The model under review builds one solid part; all positions refer to its coordinate system, in mm. Face numbers are marked on the shaded views. A direction names the side the tool comes from. Coordinates: 2 decimals unless noted, no trailing zeros. Loops run counter-clockwise (first coordinate to the right, second up) from the corner with the lowest first, then second, coordinate; pieces in that order, holes last. Notation, with made-up numbers: M -21.75,-10 L 21.25,-10 A5 cw 21.25,-4 Z; hole C 26,66 d4. An arc over 180 degrees is marked long. Use CSV: the item, a comma, the result in double quotes. Start each with the question number.
from build123d import *

# Parameters (mm, degrees)
BOSS_EXTRUDE1_DEPTH     = 24
FILLET1_R               = 14
CUT_EXTRUDE1_DEPTH      = 36
CUT_EXTRUDE1_DEPTH_BACK = 21


with BuildPart() as part:
    # Sketch1 → Boss-Extrude1 (new body, symmetric)
    with BuildSketch(Plane.XY):
        with BuildLine():
            Line((35, 0), (48, 0))
            Line((48, 0), (48, 6))
            Line((48, 6), (95, 6))
            Line((95, 6), (95, 20))
            Line((95, 20), (51.23475383, 20))
            ThreePointArc((51.23475383, 20), (0, 55), (-51.23475383, 20))
            Line((-51.23475383, 20), (-95, 20))
            Line((-95, 20), (-95, 6))
            Line((-95, 6), (-48, 6))
            Line((-48, 6), (-48, 0))
            Line((-48, 0), (-35, 0))
            ThreePointArc((-35, 0), (0, 35), (35, 0))
        make_face()
    extrude(amount=BOSS_EXTRUDE1_DEPTH, both=True)

    # Fillet1
    fillet1_edges = [part.edges().sort_by_distance(p)[0] for p in [
        (95, 13, -24),
        (-95, 13, -24),
        (95, 13, 24),
        (-95, 13, 24),
    ]]
    fillet(fillet1_edges, radius=FILLET1_R)

    # Sketch2 → Cut-Extrude1 (cut, two sides)
    with BuildSketch(Plane(origin=(0, 20, 0), x_dir=(1, 0, 0), z_dir=(0, 1, 0))) as cut_extrude1_sk:
        with BuildLine():
            Line((68, -7), (68, 13))
            ThreePointArc((68, 13), (75, 20), (82, 13))
            Line((82, 13), (82, -7))
            ThreePointArc((82, -7), (75, -14), (68, -7))
        make_face()
        with BuildLine():
            Line((-68, -7), (-68, 13))
            ThreePointArc((-68, 13), (-75, 20), (-82, 13))
            Line((-82, 13), (-82, -7))
            ThreePointArc((-82, -7), (-75, -14), (-68, -7))
        make_face()
    extrude(amount=CUT_EXTRUDE1_DEPTH, mode=Mode.SUBTRACT)
    extrude(cut_extrude1_sk.sketch, amount=-CUT_EXTRUDE1_DEPTH_BACK, mode=Mode.SUBTRACT)


solid = part.part
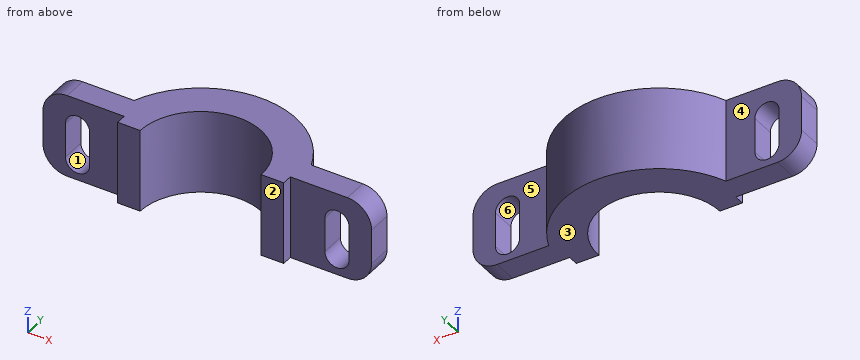
1. Add section D-D (y = 25.5). Write out the cut boundary in (x, z).
2. For the marked faces 4, 5 and 6, list the 3-axis set-ups (+Z, -Z, +X, -X, +Y, -Y) from which the entire face can be reached by the end or side of a thin tool; tool diameter is ignored.
3. Add section C-C (z = -16). Write out the cut boundary in (x, y).
4. Add section A-A (x = -75). Write out the cut boundary in (y, z), plus the area to 3 significant figures.
5. Draft analysis for pull direction Z (two halves, no side actions). For the marked faces 1, 2 and 3, state which applies: released by +Z, released by -Z, zero draft, split by the parting line, or undercut.
6. Insertion check: pin 1 Ø1 at (y, z) = (30.5, 0.5) entering from +X; pin 2 Ø1.5 at (y, z) = (37.5, -10.5) entering from -X; pin 3 Ø8 at (x, z) = (58.5, -3) entering from -Y. Each pin has a flat end and moves straight along its axis. Give the tip position at first contact, or say it passes through.
7. To check wall thickness, follow line 1 along X through (y, z) = (17.5, -2); line 2 along X through (y, z) = (15, -0.5); line 3 along Y through (x, z) = (84.5, -1). State the ranges of each line that lie inside material, in increasing order.
8. Add section B-B (y = 17). Write out the cut boundary in (x, z).
Solved:
1,outline,"M -48.73,-24 L -23.97,-24 L -23.97,24 L -48.73,24 Z; M 23.97,-24 L 48.73,-24 L 48.73,24 L 23.97,24 Z"
2,face 4,"+Z, -Z, -X, +Y"
2,face 5,"+Z, -Z, +X, +Y"
2,face 6,"+Y, -Y"
3,outline,"M -93.65,6 L -81.32,6 L -81.32,20 L -93.65,20 Z; M -68.68,6 L -48,6 L -48,0 L -35,0 A35 cw 35,0 L 48,0 L 48,6 L 68.68,6 L 68.68,20 L 51.23,20 A55 ccw -51.23,20 L -68.68,20 Z; M 81.32,6 L 93.65,6 L 93.65,20 L 81.32,20 Z"
4,outline,"M 6,-24 L 20,-24 L 20,-20 L 6,-20 Z; M 6,14 L 20,14 L 20,24 L 6,24 Z"
4,area,"196 mm^2"
5,face 1,"undercut"
5,face 2,"zero draft"
5,face 3,"released by -Z"
6,pin 1,"stops at x = 46.1"
6,pin 2,"stops at x = -40.92"
6,pin 3,"stops at y = 6"
7,line 1,"x = -95 to -82, -68 to -30.31, 30.31 to 68, 82 to 95"
7,line 2,"x = -95 to -82, -68 to -31.62, 31.62 to 68, 82 to 95"
7,line 3,"y = 6 to 20"
8,outline,"M -95,-10 A14 ccw -81,-24 L -30.59,-24 L -30.59,24 L -81,24 A14 ccw -95,10 Z; M 30.59,-24 L 81,-24 A14 ccw 95,-10 L 95,10 A14 ccw 81,24 L 30.59,24 Z; hole M -82,-13 A7 ccw -68,-13 L -68,7 A7 ccw -82,7 Z; hole M 68,-13 A7 ccw 82,-13 L 82,7 A7 ccw 68,7 Z"
